The model under review builds one solid part; all positions refer to its coordinate system, in mm. Face numbers are marked on the shaded views. A direction names the side the tool comes from. Round coordinates to 2 decimals unless told otherwise and drop trailing zeros. Order: outer loops, then holes, each group sorted by start corner. A loop starts at its lowest first (then second) coordinate and runs counter-clockwise, first axis right, second up.
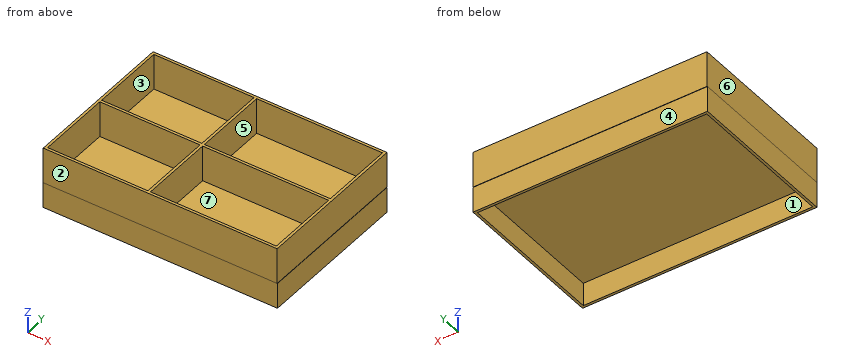
```python
from build123d import *

# Parameters (mm, degrees)
F0_W     = 455
F0_H     = 305
F0_W_2   = 195
F0_H_2   = 145
F0_W_3   = 245
F1_DEPTH = 70
F2_W     = 456.144392
F2_H     = 304.169386
F3_DEPTH = 5
F4_W     = 456.144392
F4_H     = 304.169386
F4_W_2   = 446.144392
F4_H_2   = 294.169386
F5_DEPTH = 45


with BuildPart() as f1:
    # F0 (on Top) → F1 (new body)
    with BuildSketch(Plane.XY):
        with Locations((-2.477493, -2.5)):
            Rectangle(F0_W, F0_H)
        with Locations((-127.477493, -77.5)):
            Rectangle(F0_W_2, F0_H_2, mode=Mode.SUBTRACT)
        with Locations((97.522507, -77.5)):
            Rectangle(F0_W_3, F0_H_2, mode=Mode.SUBTRACT)
        with Locations((-127.477493, 72.5)):
            Rectangle(F0_W_2, F0_H_2, mode=Mode.SUBTRACT)
        with Locations((97.522507, 72.5)):
            Rectangle(F0_W_3, F0_H_2, mode=Mode.SUBTRACT)
    extrude(amount=F1_DEPTH)

    # F2 (on face) → F3 (join)
    with BuildSketch(Plane.XY):
        with Locations((-2.442673, -2.826333)):
            Rectangle(F2_W, F2_H)
    extrude(amount=-F3_DEPTH)

    # F4 (on face) → F5 (join)
    with BuildSketch(Plane(origin=(0, 0, -5), x_dir=(1, 0, 0), z_dir=(0, 0, -1))):
        with Locations((-2.442673, 2.826333)):
            Rectangle(F4_W, F4_H)
        with Locations((-2.442673, 2.826333)):
            Rectangle(F4_W_2, F4_H_2, mode=Mode.SUBTRACT)
    extrude(amount=F5_DEPTH)


solid = f1.part
```
(1) For the marked faces 1, 2 and 3, list the 3-axis set-ups (+Z, -Z, +X, -X, +Y, -Y) from which the entire face can be reached by the end or side of a thin tool; tool diameter is ignored.
Data:
face 1: -Z
face 2: +Z, -Z, +X, -X, -Y
face 3: +Z
(2) Consider section C-C (z = 40.5). Write out the cut boundary in (x, y).
Data:
outline: (-229.98, -155) - (225.02, -155) - (225.02, 150) - (-229.98, 150) - close; hole (-224.98, -150) - (-29.98, -150) - (-29.98, -5) - (-224.98, -5) - close; hole (-224.98, 0) - (-29.98, 0) - (-29.98, 145) - (-224.98, 145) - close; hole (-24.98, -150) - (220.02, -150) - (220.02, -5) - (-24.98, -5) - close; hole (-24.98, 0) - (220.02, 0) - (220.02, 145) - (-24.98, 145) - close
(3) Consider section B-B (y = -53). Write out the cut boundary in (x, z), and give its area (3 significant figures).
Data:
outline: (-230.51, -50) - (-225.51, -50) - (-225.51, -5) - (220.63, -5) - (220.63, -50) - (225.63, -50) - (225.63, 0) - (225.02, 0) - (225.02, 70) - (220.02, 70) - (220.02, 0) - (-24.98, 0) - (-24.98, 70) - (-29.98, 70) - (-29.98, 0) - (-224.98, 0) - (-224.98, 70) - (-229.98, 70) - (-229.98, 0) - (-230.51, 0) - close
area: 3,780 mm2
(4) Consider section A-A (z = -36). Write out the cut boundary in (x, y), and give its area (3 significant figures).
Data:
outline: (-230.51, -154.91) - (225.63, -154.91) - (225.63, 149.26) - (-230.51, 149.26) - close; hole (-225.51, -149.91) - (220.63, -149.91) - (220.63, 144.26) - (-225.51, 144.26) - close
area: 7,500 mm2
(5) To check wall thickness, follow probe 1 along Y at (x, z) = (-180, 53.5); probe 2 along X at (y, z) = (-96, 38); probe 3 along X at (y, z) = (-108, -35). State the ranges of each line that lie inside material, in increasing order.
Data:
probe 1: y = -155 to -150, -5 to 0, 145 to 150
probe 2: x = -229.98 to -224.98, -29.98 to -24.98, 220.02 to 225.02
probe 3: x = -230.51 to -225.51, 220.63 to 225.63
(6) Draft analysis for pull direction X (two halves, no side actions). For the marked faces 4, 5, 6 and 7, state which applies: pulls with the +X half, pulls with the -X half, needs draft (parallel to the pull), parting line crosses it, or undercut.
Data:
face 4: needs draft
face 5: undercut
face 6: pulls with the -X half
face 7: undercut
(7) Consider section D-D (x = 124). Write out the cut boundary in (y, z), and give its area (3 significant figures).
Data:
outline: (-155, 0) - (-154.91, 0) - (-154.91, -50) - (-149.91, -50) - (-149.91, -5) - (144.26, -5) - (144.26, -50) - (149.26, -50) - (149.26, 0) - (150, 0) - (150, 70) - (145, 70) - (145, 0) - (0, 0) - (0, 70) - (-5, 70) - (-5, 0) - (-150, 0) - (-150, 70) - (-155, 70) - close
area: 3,020 mm2
(8) Insertion check: pin 1 (6 mm diameter, centred on y = -10, z = 24.5, fed in from +X); pin 2 (6 mm diameter, centred on x = 73, z = -3.5, fed in from -Y); pin 3 (13.5 mm diameter, centred on x = -62, z = -23, fed in from +Y). Each pin has a flat end and moves straight along its axis. Give the tip position at first contact, or say it passes through.
Data:
pin 1: stops at x = 225.02
pin 2: stops at y = -154.91
pin 3: stops at y = 149.26
